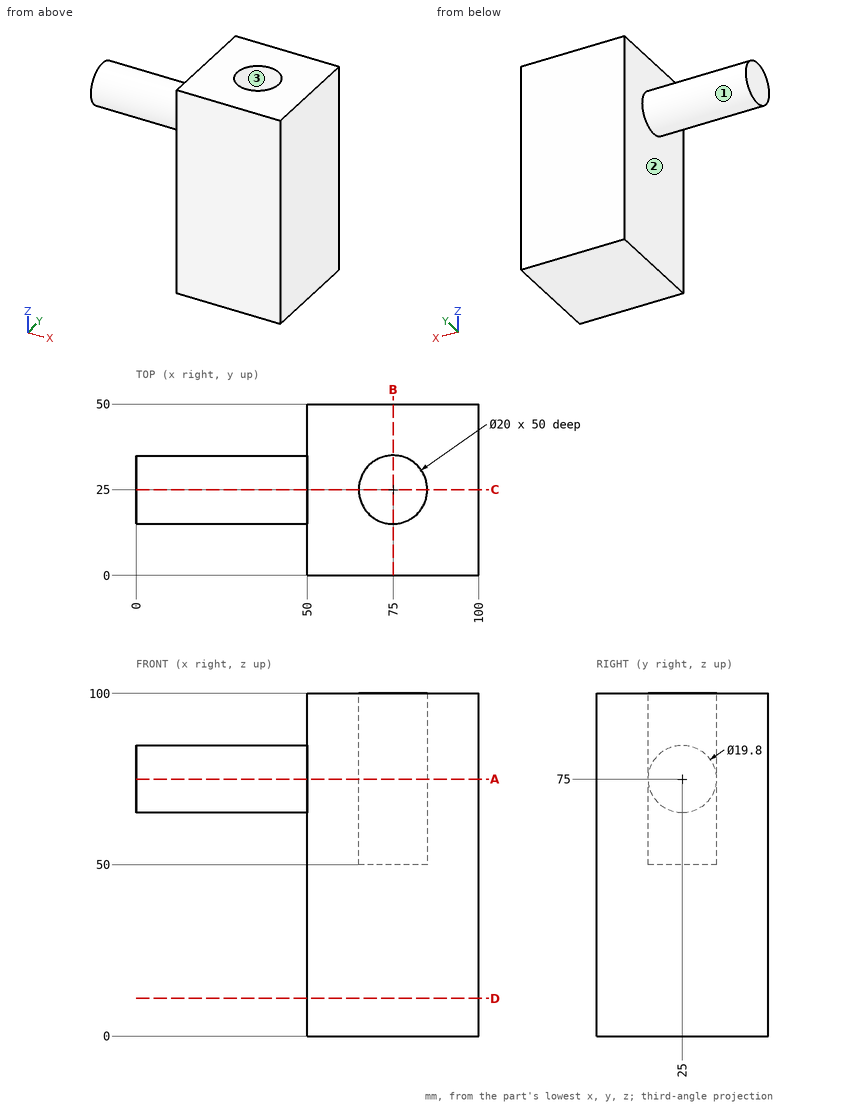
Design review of the part shown in the three views and the two pictorial views. Dimensions are in mm from the part's minimum x, y and z. Give positions to 0.01 mm unless a question says otherwise; leave off trailing zeros. Write each loop counter-clockwise with the first axis right and the second up, starting at its lowest first coordinate (ties: lowest second). Pieces come first, ordered by that corner, then holes. Notation, with made-up numbers: (37, -10) -> (67, -10) arc R15 ccw to (67, 7) -> close; hole circle Ø5 at (-12, 15). An arc over 180 degrees is marked (long way). Answer in a Markdown table with one row per item.
1) For L1, parallel to Y at x = 75, z = 89; L2, parallel to X at y = 9.5, z = 35.5; L3, parallel to Z at x = 71, y = 22, list the stretches that pass through material, from the lowest coordinate up. Write a range as [from, to].
Worked answers:
| item | result |
|---|---|
| L1 | [0, 15], [35, 50] |
| L2 | [50, 100] |
| L3 | [0, 50] |
2) Clearance check with flat-ended pins moving along their axes: P1, Ø6, axis at x = 72.5, y = 28, coming from the +Z side; P2, Ø2, axis at y = 17, z = 40.5, coming from the -X side; P3, Ø1.5, axis at x = 12, y = 12.5, coming from the +Z side (3 decimals). State where each tip first meets the part, or that it passes through.
Worked answers:
| item | result |
|---|---|
| P1 | z = 50 |
| P2 | x = 50 |
| P3 | through |
3) Mouldability with a two-part tool opening along X and no side actions: class the marked faces 1, 2 and 3 as +X half, -X half, draft (parallel to the pull), parting line (faces both ways), or undercut.
Worked answers:
| item | result |
|---|---|
| face 1 | draft |
| face 2 | -X half |
| face 3 | undercut |
4) Add section B-B on x = 75. State the section outline as (y, z) points.
Worked answers:
| item | result |
|---|---|
| outline | (0, 0) -> (50, 0) -> (50, 100) -> (35, 100) -> (35, 50) -> (15, 50) -> (15, 100) -> (0, 100) -> close |
5) Add section D-D on z = 11. State the section outline as (x, y) points.
Worked answers:
| item | result |
|---|---|
| outline | (50, 0) -> (100, 0) -> (100, 50) -> (50, 50) -> close |
6) Add section C-C on y = 25. State the section outline as (x, z) points, plus the area to 3 significant figures.
Worked answers:
| item | result |
|---|---|
| outline | (0, 65.1) -> (50, 65.1) -> (50, 0) -> (100, 0) -> (100, 100) -> (85, 100) -> (85, 50) -> (65, 50) -> (65, 100) -> (50, 100) -> (50, 84.9) -> (0, 84.9) -> close |
| area | 4,990 mm² |
7) Add section A-A on z = 75. State the section outline as (x, y) points, plus the area to 3 significant figures.
Worked answers:
| item | result |
|---|---|
| outline | (0, 15.1) -> (50, 15.1) -> (50, 0) -> (100, 0) -> (100, 50) -> (50, 50) -> (50, 34.9) -> (0, 34.9) -> close; hole circle Ø20 at (75, 25) |
| area | 3,180 mm² |
